The listing builds one solid part. Answer for the finished solid, in the listing's coordinates (mm). Face numbers are marked on the shaded views. A direction names the side the tool comes from. Coordinates: 2 decimals unless noted, no trailing zeros. Order: outer loops, then holes, each group sorted by start corner. A loop starts at its lowest first (then second) coordinate and runs counter-clockwise, first axis right, second up.
Autodesk Inventor part; units mm, degrees
ref_plane "YZ Plane" through (0, 0, 0) normal (1, 0, 0) x (0, 1, 0)
ref_plane "XZ Plane" through (0, 0, 0) normal (0, 1, 0) x (-1, 0, 0)
ref_plane "XY Plane" through (0, 0, 0) normal (0, 0, 1) x (1, 0, 0)
sketch "Skizze1" plane through (0, 0, 0) normal (0, 0, 1) x (1, 0, 0)
  line L0 (-123.0333, 0) -> (142.9667, 0)
  line L1 (0, -107.5057) -> (0, 172.4943)
  line L2 (-75.0333, 122.4943) -> (94.9667, 122.4943)
  line L3 (94.9667, 122.4943) -> (94.9667, -57.5057)
  line L4 (94.9667, -57.5057) -> (-75.0333, -57.5057)
  line L5 (-75.0333, -57.5057) -> (-75.0333, 122.4943)
  line L6 (-85.0333, 132.4943) -> (104.9667, 132.4943)
  line L7 (104.9667, 132.4943) -> (104.9667, -67.5057)
  line L8 (104.9667, -67.5057) -> (-85.0333, -67.5057)
  line L9 (-85.0333, -67.5057) -> (-85.0333, 132.4943)
  point P0 (0, 0)
  dimension "d0" = 170
  dimension "d1" = 180
  dimension "d2" = 10
  dimension "d3" = 10
  dimension "d4" = 10
  dimension "d5" = 10
extrude "Extrusion1" add sketch "Skizze1" along normal blind 100 contours L9 L6 L1 L2 L5 L0 | L0 L5 L4 L1 L8 L9 | L1 L4 L3 L0 L7 L8 | L6 L7 L0 L3 L2 L1
sketch "Skizze2" plane through (0, 0, 100) normal (0, 0, 1) x (1, 0, 0)
  point P0 (0, 0)
sketch "Skizze3" plane through (0, 0, 100) normal (0, 0, 1) x (1, 0, 0)
  line L0 (-85.0333, 132.4943) -> (-85.0333, -67.5057)
  line L1 (-85.0333, 132.4943) -> (104.9667, 132.4943)
  line L2 (104.9667, 132.4943) -> (104.9667, -67.5057)
  line L3 (104.9667, -67.5057) -> (-85.0333, -67.5057)
  line L4 (-85.0333, -67.5057) -> (-85.0333, 132.4943)
  point P0 (0, 0)
extrude "Extrusion2" add sketch "Skizze3" along normal blind 50
fillet "Rundung1" radius 92 4 edges at (-85.0333, 32.4943, 150) (9.9667, 132.4943, 150) (9.9667, -67.5057, 150) (104.9667, 32.4943, 150)
sketch "Skizze4" plane through (0, 0, 150) normal (0, 0, 1) x (1, 0, 0)
  point P0 (0, 0)
sketch "Skizze5" plane through (0, 0, 150) normal (0, 0, 1) x (1, 0, 0)
  line L0 (6.9667, 24.4943) -> (6.9667, 40.4943)
  line L1 (94.8203, -57.3593) -> (12.9667, 24.4943)
  line L2 (6.9667, 40.4943) -> (12.9667, 40.4943)
  line L3 (12.9667, 40.4943) -> (12.9667, 24.4943)
  line L4 (12.9667, 24.4943) -> (6.9667, 24.4943)
  line L5 (6.9667, 24.4943) -> (6.9667, 40.4943)
  point P0 (0, 0)
extrude "Extrusion3" cut sketch "Skizze5" against normal blind 50
properties part number "Deckel" material "PMMA-Kunststoff"
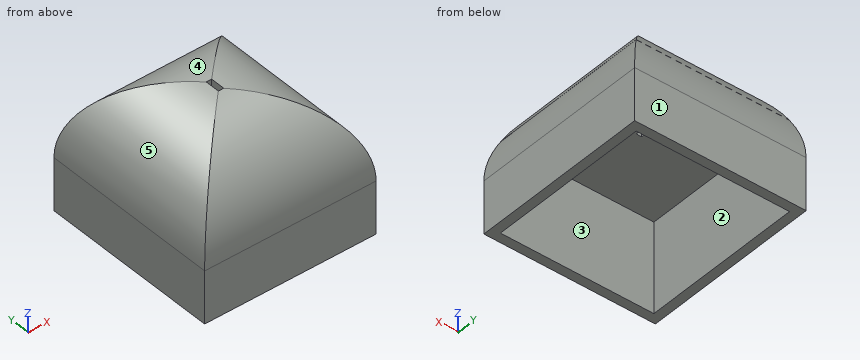
(1) Find the intervals of material crossed by probe 1 along X at (y, z) = (24, 42.5); probe 2 along Y at (x, z) = (-71, 14); probe 3 along X at (y, z) = (39, 95), in increasing order.
(2) The mould has two halves that part along X. Classify the marked faces 3, 4 and 5: pulls with the +X half, pulls with the -X half, needs draft (parallel to the pull), parting line crosses it, or undercut.
(3) Find section A-A on z = 35. Determine the outline of the cut face in (x, y).
(4) Find section D-D on z = 115. Determine the outline of the cut face in (x, y).
(5) Given pin 1 Ø1.5 at (x, y) = (-48.5, 18.5) entering from -Z; pin 2 Ø5 at (x, z) = (11, 133) entering from -Y; pin 3 Ø6 at (x, z) = (21.5, 95.5) entering from -Y, each flat-ended and moving along its own axis, determine where each tip first touches the part or whether it passes through.
(6) A tool of negligible diameter and unlimited length cuts with its end or side. For the marked faces 1 and 2, from which of +Z, -Z, +X, -X, +Y, -Y can it reach the whole face along a straight path? Write none if from no direction.
Resolved:
1. probe 1: x = -85.03 to -75.03, 94.97 to 104.97
1. probe 2: y = -67.51 to -57.51, 122.49 to 132.49
1. probe 3: x = -77.27 to -75.03, 94.97 to 97.2
2. face 3: undercut
2. face 4: needs draft
2. face 5: pulls with the -X half
3. outline: (-85.03, -67.51) - (104.97, -67.51) - (104.97, 132.49) - (-85.03, 132.49) - close; hole (-75.03, -57.51) - (94.97, -57.51) - (94.97, 122.49) - (-75.03, 122.49) - close
4. outline: (-65.25, -47.72) - (85.18, -47.72) - (85.18, 112.71) - (-65.25, 112.71) - close; hole (6.97, 24.49) - (12.97, 24.49) - (12.97, 40.49) - (6.97, 40.49) - close
5. pin 1: stops at z = 100
5. pin 2: stops at y = -32.14
5. pin 3: stops at y = -60.79
6. face 1: +Z, -Z, +X, -X, +Y
6. face 2: -Z
